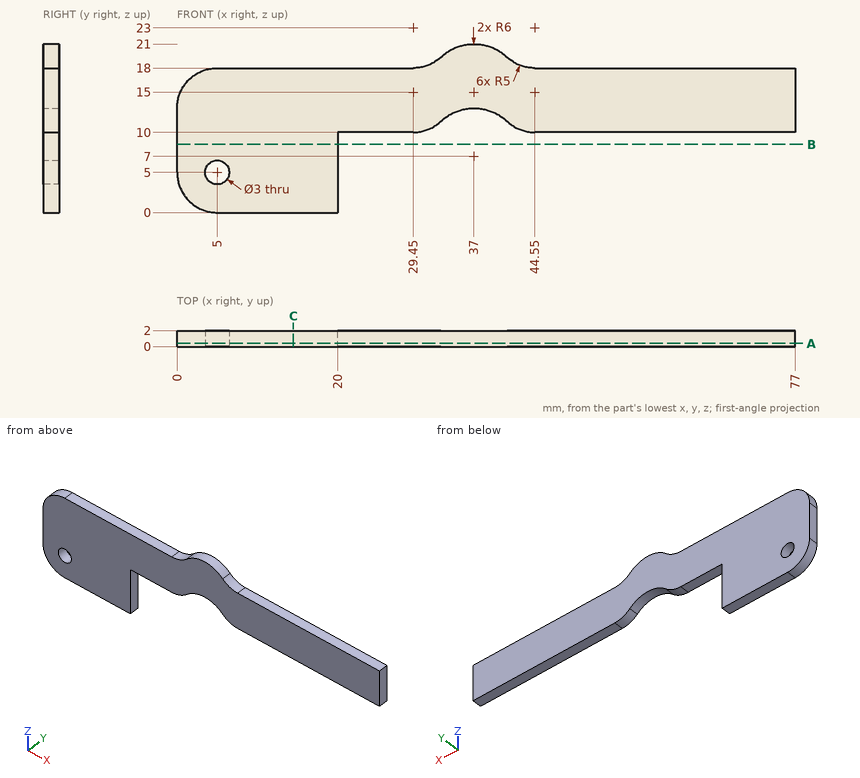
Geometry: see drawing. Coordinates: mm, zero at the bounding-box minimum. Give positions to 0.01 mm unless a question says otherwise; leave off trailing zeros. Order: outer loops, then holes, each group sorted by start corner. A loop starts at its lowest first (then second) coordinate and runs counter-clockwise, first axis right, second up.
Q1. Section C-C on x = 14.5. Output: boundary loops of the cut face in (y, z), and give its area (3 significant figures).
Checked values:
outline: (0, 0) - (2, 0) - (2, 18) - (0, 18) - close
area: 36.0 mm2
Q2. Section B-B on z = 8.5. Output: boundary loops of the cut face in (x, y).
Checked values:
outline: (0, 0) - (20, 0) - (20, 2) - (0, 2) - close
Q3. Section A-A on y = 0.4. Output: boundary loops of the cut face in (x, z).
Checked values:
outline: (0, 5) arc R5 ccw to (5, 0) - (20, 0) - (20, 10) - (29.45, 10) arc R5 ccw to (32.88, 11.36) arc R6 cw to (41.12, 11.36) arc R5 ccw to (44.55, 10) - (77, 10) - (77, 18) - (44.55, 18) arc R5 cw to (41.12, 19.36) arc R6 ccw to (32.88, 19.36) arc R5 cw to (29.45, 18) - (5, 18) arc R5 ccw to (0, 13) - close; hole circle Ø3 at (5, 5)
Q4. Ray query, probe 1 along X at (y, z) = (1.05, 5); probe 2 along Z at (x, y) = (13, 0.25); probe 3 along Z at (x, y) = (67.5, 1.05). Return the intervals inside material, ascending.
Checked values:
probe 1: x = 0 to 3.5, 6.5 to 20
probe 2: z = 0 to 18
probe 3: z = 10 to 18
Q5. Contact query for flat-ended pins moving along their axis: pin 1 Ø0.6 at (x, y) = (13.5, 1) entering from +Z; pin 2 Ø0.6 at (x, y) = (58, 1.5) entering from -Z; pin 3 Ø0.6 at (y, z) = (1, 6) entering from +X. Output: stop coordinate, or through.
Checked values:
pin 1: stops at z = 18
pin 2: stops at z = 10
pin 3: stops at x = 20
